Build history of the part. All positions in model axes, mm. A direction names the side the tool comes from. Give positions to 0.01 mm unless a question says otherwise; leave off trailing zeros. Order: outer loops, then holes, each group sorted by start corner. A loop starts at its lowest first (then second) coordinate and runs counter-clockwise, first axis right, second up. Notation, with made-up numbers: M 55.5,-20 L 95.5,-20 A23 cw 95.5,-1 Z; hole C -30,42.25 d10. An arc over 180 degrees is marked long. Use CSV: the item, a comma, the result in double quotes. Start each with the question number.
Item 1: Wall check: line 1 along Z through (x, y) = (23, 1.2); line 2 along X through (y, z) = (0.9, -35); line 3 along X through (y, z) = (-6, 24) (3 decimals). Give the ranges that are in metal, low to high.
Item 2: Band-saw the part on D-D on z = 35. Write the cut outline in (x, y), plus the area to 3 significant figures.
Item 3: Which spindle directions (+Z, -Z, +X, -X, +Y, -Y) get a long thin tool onto all of the face, cutting with end or side? Do faces 1 (the flat face through (-25, -3, -27)), 2 (the flat face through (-10, 1, 40)), 3 (the flat face through (-25, -1, 25.5)). Say none if no direction does.
Item 4: Pin check, flat tips, straight feed: P1, Ø1.5, axis at x = -36.5, y = -2, coming from the +Z side; P2, Ø4, axis at y = -3.5, z = 2.5, coming from the +X side (3 decimals); P3, Ø4, axis at x = 3, z = -0.5, coming from the -Y side. Stop position of each tip, or through.
Item 5: Two-plate mould, pull along Z, no slides. Class faces 4 (the flat face through (4.925, -5, 0)), 5 (the flat face through (2, -7, 27.82)), 6 (the flat face through (2, -10, -20)): pulls with the +Z half, pulls with the -Z half, needs draft (parallel to the pull), parting line crosses it, or undercut.
Item 6: Band-saw the part on C-C on z = 14. Write the cut outline in (x, y) (3 decimals).
Item 7: Band-saw the part on A-A on x = 23. Write the cut outline in (y, z), plus the area to 3 significant figures.
Item 8: Band-saw the part on B-B on y = -10. Write the cut outline in (x, z) (3 decimals).
from build123d import *

# Parameters (mm, degrees)
A_BASE_T42_OUTLINE_R          = 2.2479
A_BASE_T42_OUTLINE_R_2        = 1
A_BASE_T42_DEPTH              = 3
OUTER_RIM_CUT_DEPTH           = 68.299702823
SKETCH2_W                     = 20
SKETCH2_H                     = 3
FLANGES_DEPTH                 = 3
CONTOURING_R                  = 1
SKETCH9_R                     = 1
SINGLE_TENDON_PORT_DEPTH      = 65.986537067
SKETCH3_W                     = 15
SKETCH3_H                     = 3
SKETCH3_W_2                   = 3
SKETCH3_H_2                   = 15
BASE_SUPPORTS_DEPTH           = 3
BASE_SUPPORTS_CHAMFER_SIZE    = 3
SKETCH10_R                    = 1
COVER_DEPTH                   = 3
SKETCH6_W                     = 5
SKETCH6_H                     = 55.64
SERVO_SIDE_SUPPORTS_DEPTH     = 8.5
SKETCH7_W                     = 5
SKETCH7_H                     = 7.82
SERVO_SIDE_SUPPORT_ENDS_DEPTH = 5
SERVO_CONTOURING_R            = 1


with BuildPart() as part:
    # a_base_t42: read off the stored shape, not the designer's step
    # a_base_t42 outline → a_base_t42 (new body)
    with BuildSketch(Plane(origin=(0, 0, 0), x_dir=(1, 0, 0), z_dir=(0, 1, 0))):
        with BuildLine():
            ThreePointArc((31.5, -42), (52.5, 0), (31.5, 42))
            Line((31.5, 42), (-31.5, 42))
            ThreePointArc((-31.5, 42), (-52.5, 0), (-31.5, -42))
            Line((-31.5, -42), (31.5, -42))
        make_face()
        with Locations((-23, -35)):
            Circle(A_BASE_T42_OUTLINE_R, mode=Mode.SUBTRACT)
        with Locations((23, -35)):
            Circle(A_BASE_T42_OUTLINE_R, mode=Mode.SUBTRACT)
        with Locations((-40.25, 0)):
            Circle(A_BASE_T42_OUTLINE_R_2, mode=Mode.SUBTRACT)
        with Locations((-23, 35)):
            Circle(A_BASE_T42_OUTLINE_R, mode=Mode.SUBTRACT)
        with Locations((40.25, 0)):
            Circle(A_BASE_T42_OUTLINE_R_2, mode=Mode.SUBTRACT)
        with Locations((23, 35)):
            Circle(A_BASE_T42_OUTLINE_R, mode=Mode.SUBTRACT)
    extrude(amount=A_BASE_T42_DEPTH)

    # Sketch1 → Outer Rim Cut (cut, through all)
    with BuildSketch(Plane.XZ):
        with BuildLine():
            Line((31.5, 42), (-31.5, 42))
            ThreePointArc((-31.5, 42), (-52.5, 0), (-31.5, -42))
            Line((-31.5, -42), (31.5, -42))
            ThreePointArc((31.5, -42), (52.5, 0), (31.5, 42))
        make_face()
        with BuildLine():
            Line((30.483602149, 39), (-30.483602149, 39))
            ThreePointArc((-30.483602149, 39), (-49.5, 0), (-30.483602149, -39))
            Line((-30.483602149, -39), (30.483602149, -39))
            ThreePointArc((30.483602149, -39), (49.5, 0), (30.483602149, 39))
        make_face(mode=Mode.SUBTRACT)
    extrude(amount=-OUTER_RIM_CUT_DEPTH, mode=Mode.SUBTRACT)

    # Sketch2 → Flanges (add)
    with BuildSketch(Plane.XZ):
        with Locations((0, -40.5)):
            Rectangle(SKETCH2_W, SKETCH2_H)
        with Locations((0, 40.5)):
            Rectangle(SKETCH2_W, SKETCH2_H)
    extrude(amount=-FLANGES_DEPTH)

    # Contouring
    contouring_edges = [part.edges().sort_by_distance(p)[0] for p in [
        (30.483602149, 1.5, -39),
        (-30.483602149, 1.5, -39),
        (10, 1.5, -42),
        (-10, 1.5, -42),
        (30.483602149, 1.5, 39),
        (-30.483602149, 1.5, 39),
        (10, 1.5, 42),
        (-10, 1.5, 42),
    ]]
    fillet(contouring_edges, radius=CONTOURING_R)

    # Sketch9 → Single Tendon Port (cut, through all)
    with BuildSketch(Plane.XZ):
        with Locations(Location((11.425, 0, 0), (0, 0, 270))):
            Circle(SKETCH9_R)
    extrude(amount=-SINGLE_TENDON_PORT_DEPTH, mode=Mode.SUBTRACT)

    # Sketch3 → Base Supports (add)
    with BuildSketch(Plane.XZ):
        with Locations((-25.325, -27)):
            Rectangle(SKETCH3_W, SKETCH3_H)
        with Locations((-25.325, 27)):
            Rectangle(SKETCH3_W, SKETCH3_H)
        with Locations((-34.325, -12.5)):
            Rectangle(SKETCH3_W_2, SKETCH3_H_2)
        with Locations((-34.325, 12.5)):
            Rectangle(SKETCH3_W_2, SKETCH3_H_2)
    extrude(amount=BASE_SUPPORTS_DEPTH)

    # Base Supports Chamfer
    # the kernel refuses this chamfer: 3 mm, written as the material it adds along each edge
    with BuildSketch(Plane(origin=(-32.825, 0, 28.5), x_dir=(0, 0, 1), z_dir=(1, 0, 0))) as base_supports_chamfer_piece_1_section:
        Polygon((BASE_SUPPORTS_CHAMFER_SIZE, 0), (0, BASE_SUPPORTS_CHAMFER_SIZE), (0, 0), align=None)
    base_supports_chamfer_piece_1 = extrude(amount=15, mode=Mode.PRIVATE)
    base_supports_chamfer_piece_1 = split(base_supports_chamfer_piece_1, bisect_by=Plane(origin=(-32.825, -3, 28.5), z_dir=(0, 1, 0)), keep=Keep.TOP, mode=Mode.PRIVATE)
    add(base_supports_chamfer_piece_1)
    with BuildSketch(Plane(origin=(-17.825, 0, -28.5), x_dir=(0, 0, -1), z_dir=(-1, 0, 0))) as base_supports_chamfer_piece_2_section:
        Polygon((BASE_SUPPORTS_CHAMFER_SIZE, 0), (0, BASE_SUPPORTS_CHAMFER_SIZE), (0, 0), align=None)
    base_supports_chamfer_piece_2 = extrude(amount=15, mode=Mode.PRIVATE)
    base_supports_chamfer_piece_2 = split(base_supports_chamfer_piece_2, bisect_by=Plane(origin=(-17.825, -3, -28.5), z_dir=(0, 1, 0)), keep=Keep.TOP, mode=Mode.PRIVATE)
    add(base_supports_chamfer_piece_2)
    with BuildSketch(Plane(origin=(-35.825, 0, 20), x_dir=(-1, 0, 0), z_dir=(0, 0, -1))) as base_supports_chamfer_piece_3_section:
        Polygon((BASE_SUPPORTS_CHAMFER_SIZE, 0), (0, -BASE_SUPPORTS_CHAMFER_SIZE), (0, 0), align=None)
    base_supports_chamfer_piece_3 = extrude(amount=15, mode=Mode.PRIVATE)
    base_supports_chamfer_piece_3 = split(base_supports_chamfer_piece_3, bisect_by=Plane(origin=(-35.825, -3, 20), z_dir=(0, 1, 0)), keep=Keep.TOP, mode=Mode.PRIVATE)
    add(base_supports_chamfer_piece_3)
    with BuildSketch(Plane(origin=(-35.825, 0, -20), x_dir=(-1, 0, 0), z_dir=(0, 0, 1))) as base_supports_chamfer_piece_4_section:
        Polygon((BASE_SUPPORTS_CHAMFER_SIZE, 0), (0, BASE_SUPPORTS_CHAMFER_SIZE), (0, 0), align=None)
    base_supports_chamfer_piece_4 = extrude(amount=15, mode=Mode.PRIVATE)
    base_supports_chamfer_piece_4 = split(base_supports_chamfer_piece_4, bisect_by=Plane(origin=(-35.825, -3, -20), z_dir=(0, 1, 0)), keep=Keep.TOP, mode=Mode.PRIVATE)
    add(base_supports_chamfer_piece_4)

    # Sketch10 → Cover (add)
    with BuildSketch(Plane.XZ):
        with Locations((-40.25, 0)):
            Circle(SKETCH10_R)
        with Locations((40.25, 0)):
            Circle(SKETCH10_R)
    extrude(amount=-COVER_DEPTH)

    # Sketch6 → Servo Side Supports (add)
    with BuildSketch(Plane.XZ):
        with Locations((2.425, 0)):
            Rectangle(SKETCH6_W, SKETCH6_H)
    extrude(amount=SERVO_SIDE_SUPPORTS_DEPTH)

    # Sketch7 → Servo Side Support Ends (add)
    with BuildSketch(Plane.XZ.offset(8.5)):
        with Locations((2.425, 23.91)):
            Rectangle(SKETCH7_W, SKETCH7_H)
        with Locations((2.425, -23.91)):
            Rectangle(SKETCH7_W, SKETCH7_H)
    extrude(amount=SERVO_SIDE_SUPPORT_ENDS_DEPTH)

    # Servo Contouring
    servo_contouring_edges = [part.edges().sort_by_distance(p)[0] for p in [
        (2.425, 0, -27.82),
        (2.425, 0, 27.82),
        (2.425, -13.5, 20),
        (2.425, -13.5, 27.82),
        (2.425, -13.5, -27.82),
        (2.425, -13.5, -20),
    ]]
    fillet(servo_contouring_edges, radius=SERVO_CONTOURING_R)


solid = part.part
Model answer:
1,line 1,"z = -39 to -37.25, -32.75 to 32.75, 37.25 to 39"
1,line 2,"x = -35 to -25.25, -20.75 to 20.75, 25.25 to 35"
1,line 3,"x = -0.075 to 4.925"
2,outline,"M -35,0 L -25.25,0 L -25.25,3 L -35,3 Z; M -20.75,0 L 20.75,0 L 20.75,3 L -20.75,3 Z; M 25.25,0 L 35,0 L 35,3 L 25.25,3 Z"
2,area,"183 mm^2"
3,face 1,"+Z, -Z, -X, -Y"
3,face 2,"+Z, -X, +Y, -Y"
3,face 3,"-X, -Y"
4,P1,"stops at z = 20"
4,P2,"stops at x = 4.925"
4,P3,"stops at y = -8.5"
5,face 4,"needs draft"
5,face 5,"pulls with the +Z half"
5,face 6,"undercut"
6,outline,"M -47.479,0 L -38.825,0 L -35.825,-3 L -32.825,-3 L -32.825,0 L -0.075,0 L -0.075,-8.5 L 4.925,-8.5 L 4.925,0 L 47.479,0 L 47.479,3 L -47.479,3 Z"
7,outline,"M 0,-39 L 3,-39 L 3,-37.25 L 0,-37.25 Z; M 0,-32.75 L 3,-32.75 L 3,32.75 L 0,32.75 Z; M 0,37.25 L 3,37.25 L 3,39 L 0,39 Z"
7,area,"207 mm^2"
8,outline,"M -0.075,-27.82 L 4.925,-27.82 L 4.925,-20 L -0.075,-20 Z; M -0.075,20 L 4.925,20 L 4.925,27.82 L -0.075,27.82 Z"
